Read the model definition and answer for the solid it produces. Units are mm, in the model's axes. Face numbers are marked on the shaded views. A direction names the side the tool comes from. Coordinates: 2 decimals unless noted, no trailing zeros. Loops run counter-clockwise (first coordinate to the right, second up) from the corner with the lowest first, then second, coordinate; pieces in that order, holes last. Notation, with made-up numbers: (-19, 38) -> (-8, 38) arc R27 cw to (-8, 69) -> close; hole circle Ø11 at (41.25, 61.5). An arc over 180 degrees is marked (long way). Answer as a JSON object with one key per item and string values. Group by question number.
Q1. Straight lines are drawn through the part: line 1 along X through (y, z) = (10.5, 27); line 2 along Z through (x, y) = (-3.5, 10); line 3 along Z through (x, y) = (2, 11). For each, find the intervals that lie inside material, in ascending order. Write a range as [from, to].
Q2. The part is cut by section B-B on x = -22. Write down the section's boundary in (y, z), and give its area (3 significant figures).
Q3. The part is cut by section A-A on y = 23. Write down the section's boundary in (x, z), and give its area (3 significant figures).
Q4. Each of these flat-tipped pins is pushed along its axis until it touches: P1, Ø2, axis at x = 16, z = 0, coming from the +Y side; P2, Ø1.5, axis at x = 21, z = -1.5, coming from the +Y side. Where does it stop, or does it pass through?
Q5. The part is cut by section C-C on z = 35.5. Write down the section's boundary in (x, y), and give its area (3 significant figures).
Q6. Determine the mould class of the marked faces 3, 4, 5 and 6 for opening direction X: released by +X, released by -X, zero draft, split by the parting line, or undercut.
Q7. For the marked faces 1 and 2, determine the directions among +Z, -Z, +X, -X, +Y, -Y from which every point of the face is accessible in a straight line to the end or side of a thin tool.
from build123d import *

# Parameters (mm, degrees)
SKETCH1_W           = 60
SKETCH1_H           = 60
BOSS_EXTRUDE1_DEPTH = 35
SKETCH2_W           = 43.4
SKETCH2_H           = 43.4
CUT_EXTRUDE1_DEPTH  = 32
SKETCH3_W           = 1.5
SKETCH3_H           = 4
CUT_EXTRUDE4_DEPTH  = 32
SKETCH7_W           = 3.5
SKETCH7_H           = 3.5
CUT_EXTRUDE7_DEPTH  = 76
BOSS_EXTRUDE4_DEPTH = 8.3
BOSS_EXTRUDE5_DEPTH = 8.3
SKETCH13_W          = 3
SKETCH13_H          = 3
CUT_EXTRUDE8_DEPTH  = 8.3
SKETCH15_W          = 3
SKETCH15_H          = 1.2
CUT_EXTRUDE9_DEPTH  = 10
SKETCH18_W          = 8.3
SKETCH18_H          = 3
BOSS_EXTRUDE7_DEPTH = 1.2
SKETCH19_W          = 5
SKETCH19_H          = 5
CUT_EXTRUDE10_DEPTH = 11.2


with BuildPart() as part:
    # Sketch1 → Boss-Extrude1 (new body)
    with BuildSketch(Plane(origin=(0, 0, 0), x_dir=(1, 0, 0), z_dir=(0, 1, 0))):
        with Locations((-4.265402844, -11.303317536)):
            Rectangle(SKETCH1_W, SKETCH1_H)
    extrude(amount=BOSS_EXTRUDE1_DEPTH)

    # Sketch2 → Cut-Extrude1 (cut)
    with BuildSketch(Plane(origin=(0, 35, 0), x_dir=(1, 0, 0), z_dir=(0, 1, 0))):
        with Locations((-4.265402844, -11.303317536)):
            Rectangle(SKETCH2_W, SKETCH2_H)
    extrude(amount=-CUT_EXTRUDE1_DEPTH, mode=Mode.SUBTRACT)

    # Sketch3 → Cut-Extrude4 (cut)
    with BuildSketch(Plane(origin=(0, 3, 0), x_dir=(1, 0, 0), z_dir=(0, 1, 0))):
        with Locations((1.484597156, 12.396682464)):
            Rectangle(SKETCH3_W, SKETCH3_H)
        with Locations((1.484597156, -35.003317536)):
            Rectangle(SKETCH3_W, SKETCH3_H)
    extrude(amount=CUT_EXTRUDE4_DEPTH, mode=Mode.SUBTRACT)

    # Sketch7 → Cut-Extrude7 (cut)
    with BuildSketch(Plane.ZY.offset(34.265402844)):
        with Locations((-5.246682464, 30.75)):
            Rectangle(SKETCH7_W, SKETCH7_H)
    extrude(amount=-CUT_EXTRUDE7_DEPTH, mode=Mode.SUBTRACT)

    # Sketch9 → Boss-Extrude4 (add)
    with BuildSketch(Plane(origin=(25.734597156, 0, 0), x_dir=(0, 0, -1), z_dir=(1, 0, 0))):
        Polygon((3.496682464, 33.408360871), (7.381092644, 33.408360871), (7.381092644, 28.341399858), (2.785501873, 28.341399858), (2.785501873, 33.408360871), align=None)
    extrude(amount=-BOSS_EXTRUDE4_DEPTH)

    # Sketch12 → Boss-Extrude5 (add)
    with BuildSketch(Plane.ZY.offset(34.265402844)):
        Polygon((-6.996682464, 33.539678427), (-3.311731013, 33.539678427), (-3.311731013, 28.43958096), (-8.388325726, 28.43958096), (-8.388325726, 33.539678427), align=None)
    extrude(amount=-BOSS_EXTRUDE5_DEPTH)

    # Sketch13 → Cut-Extrude8 (cut)
    with BuildSketch(Plane(origin=(25.734597156, 0, 0), x_dir=(0, 0, -1), z_dir=(1, 0, 0))):
        with Locations((1.396682464, 32.3)):
            Rectangle(SKETCH13_W, SKETCH13_H)
    extrude(amount=-CUT_EXTRUDE8_DEPTH, mode=Mode.SUBTRACT)

    # Sketch15 → Cut-Extrude9 (cut)
    with BuildSketch(Plane(origin=(25.734597156, 0, 0), x_dir=(0, 0, -1), z_dir=(1, 0, 0))):
        with Locations((1.396682464, 34.4)):
            Rectangle(SKETCH15_W, SKETCH15_H)
    extrude(amount=-CUT_EXTRUDE9_DEPTH, mode=Mode.SUBTRACT)

    # Sketch18 → Boss-Extrude7 (add)
    with BuildSketch(Plane(origin=(0, 30.8, 0), x_dir=(1, 0, 0), z_dir=(0, 1, 0))):
        with Locations((21.584597156, 1.396682464)):
            Rectangle(SKETCH18_W, SKETCH18_H)
    extrude(amount=BOSS_EXTRUDE7_DEPTH)

    # Sketch19 → Cut-Extrude10 (cut)
    with BuildSketch(Plane.ZY.offset(34.265402844)):
        with Locations((11.303317536, 32.5)):
            Rectangle(SKETCH19_W, SKETCH19_H)
    extrude(amount=-CUT_EXTRUDE10_DEPTH, mode=Mode.SUBTRACT)


solid = part.part
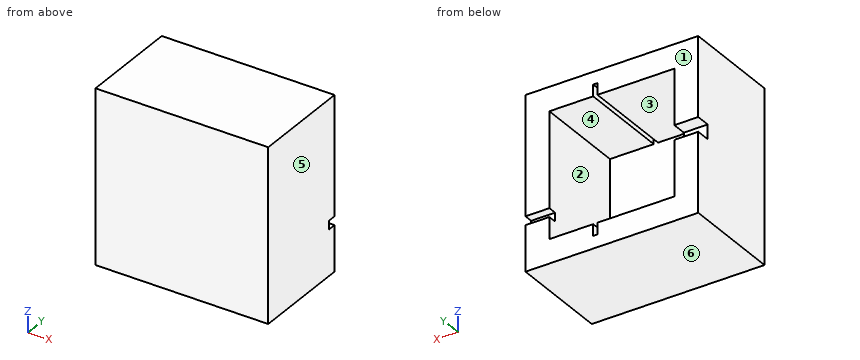
Final values:
{
 "1": {"line 1": "x = [-34.27, -25.97], [17.43, 25.73]", "line 2": "z = [-18.7, -10.4], [33, 41.3]", "line 3": "z = [-18.7, -14.4], [37, 41.3]"},
 "2": {"outline": "(0, -18.7) -> (35, -18.7) -> (35, -10.4) -> (3, -10.4) -> (3, 33) -> (35, 33) -> (35, 41.3) -> (0, 41.3) -> close", "area": "711 mm2"},
 "3": {"outline": "(-34.27, -18.7) -> (25.73, -18.7) -> (25.73, 41.3) -> (-34.27, 41.3) -> close; hole (-25.97, -10.4) -> (0.73, -10.4) -> (0.73, -14.4) -> (2.23, -14.4) -> (2.23, -10.4) -> (17.43, -10.4) -> (17.43, 33) -> (2.23, 33) -> (2.23, 37) -> (0.73, 37) -> (0.73, 33) -> (-25.97, 33) -> close", "area": "1,700 mm2"},
 "4": {"P1": "stops at y = 3", "P2": "stops at y = 32"},
 "5": {"outline": "(-34.27, 0) -> (25.73, 0) -> (25.73, 35) -> (2.23, 35) -> (2.23, 3) -> (0.73, 3) -> (0.73, 35) -> (-34.27, 35) -> close", "area": "2,050 mm2"},
 "6": {"face 3": "undercut", "face 4": "undercut", "face 5": "released by +X", "face 6": "zero draft"},
 "7": {"face 1": "+Z, -Z, +X, -X, +Y", "face 2": "+Y"}
}
